Input: part model. Units: mm. Frame: model coordinates. A direction names the side the tool comes from. Round coordinates to 2 decimals unless told otherwise and drop trailing zeros. Order: outer loops, then holes, each group sorted by start corner. A loop starts at its lowest first (then second) coordinate and runs counter-clockwise, first axis right, second up.
Item 1: Cut plane A-A on x = 12. Output: boundary loops of the cut face in (y, z), then the cut area to 4 significant figures.
Item 2: Cut plane B-B on z = 0. Output: boundary loops of the cut face in (x, y), then the cut area to 3 significant figures.
Item 3: First-contact query: pin 1 (3 mm diameter, centred on x = -15.5, z = -5.5, fed in from +Y); pin 2 (4 mm diameter, centred on x = 4, z = -9, fed in from -Y). Flat tips, straight axial feed; report the tip coordinate or a pass-through.
Item 4: Reachability of faces 1 (the cylindrical face through (5.166, -17.76, -1.517)), 2 (the flat face through (12, -18.5, 0)), 3 (the cylindrical face through (1.26, 18.23, -2.38)) from +Z, -Z, +X, -X, +Y, -Y: full face, straight path, thin tool, end or side. Return the list, or none.
Item 5: Cut plane D-D on z = 9.5. Output: boundary loops of the cut face in (x, y), then the cut area to 3 significant figures.
Item 6: Line query: L1, parallel to Y at x = -12.5, z = -8.75; L2, parallel to Y at x = 10, z = -7. Output: solid intervals per line, ascending.
Item 7: Cut plane C-C on x = -13. Output: boundary loops of the cut face in (y, z).
```python
from build123d import *

# Parameters (mm, degrees)
HOUSING_START = -17
HOUSING_DEPTH = 34
HORN_START    = 17
SK_2_R        = 11
HORN_DEPTH    = 2.5
IDLER_START   = -18.5
SK_3_R        = 7
IDLER_DEPTH   = 1.5


with BuildPart() as part:
    # SK_1 → Housing (new body)
    with BuildSketch(Plane(origin=(0, 0, 0), x_dir=(1, 0, 0), z_dir=(0, 1, 0)).offset(HOUSING_START)):
        with BuildLine():
            Line((-21.25, -14.25), (21.25, -14.25))
            ThreePointArc((21.25, -14.25), (22.664213562, -13.664213562), (23.25, -12.25))
            Line((23.25, -12.25), (23.25, 12.25))
            ThreePointArc((23.25, 12.25), (22.664213562, 13.664213562), (21.25, 14.25))
            Line((21.25, 14.25), (-21.25, 14.25))
            ThreePointArc((-21.25, 14.25), (-22.664213562, 13.664213562), (-23.25, 12.25))
            Line((-23.25, 12.25), (-23.25, -12.25))
            ThreePointArc((-23.25, -12.25), (-22.664213562, -13.664213562), (-21.25, -14.25))
        make_face()
    extrude(amount=HOUSING_DEPTH)

    # SK_2 → Horn (add)
    with BuildSketch(Plane(origin=(0, 0, 0), x_dir=(1, 0, 0), z_dir=(0, 1, 0)).offset(HORN_START)):
        with Locations(Location((12, 0, 0), (0, 0, 270))):
            Circle(SK_2_R)
    extrude(amount=HORN_DEPTH)

    # SK_3 → Idler (add)
    with BuildSketch(Plane(origin=(0, 0, 0), x_dir=(1, 0, 0), z_dir=(0, 1, 0)).offset(IDLER_START)):
        with Locations(Location((12, 0, 0), (0, 0, 270))):
            Circle(SK_3_R)
    extrude(amount=IDLER_DEPTH)


solid = part.part
```
From the geometry:
1. outline: (-18.5, -7) - (-17, -7) - (-17, -14.25) - (17, -14.25) - (17, -11) - (19.5, -11) - (19.5, 11) - (17, 11) - (17, 14.25) - (-17, 14.25) - (-17, 7) - (-18.5, 7) - close
1. area: 1,045 mm2
2. outline: (-23.25, -17) - (5, -17) - (5, -18.5) - (19, -18.5) - (19, -17) - (23.25, -17) - (23.25, 17) - (23, 17) - (23, 19.5) - (1, 19.5) - (1, 17) - (-23.25, 17) - close
2. area: 1,660 mm2
3. pin 1: stops at y = 17
3. pin 2: stops at y = -17
4. face 1: -Y
4. face 2: +Z, -Z, +X, -X, -Y
4. face 3: +Y
5. outline: (-23.25, -17) - (23.25, -17) - (23.25, 17) - (17.55, 17) - (17.55, 19.5) - (6.45, 19.5) - (6.45, 17) - (-23.25, 17) - close
5. area: 1,610 mm2
6. L1: y = -17 to 17
6. L2: y = -17 to 19.5
7. outline: (-17, -14.25) - (17, -14.25) - (17, 14.25) - (-17, 14.25) - close
